```python
from build123d import *

# Parameters (mm, degrees)
F1_W     = 5.8
F1_H     = 2
F1_W_2   = 2
F2_DEPTH = 9
F3_DEPTH = 25
F4_R     = 1
F6_DEPTH = 7


with BuildPart() as f2:
    # F1 (on Top) → F2 (new body, symmetric)
    with BuildSketch(Plane.XY):
        with Locations((22.9, 1)):
            Rectangle(F1_W, F1_H)
        with Locations((26.8, 1)):
            Rectangle(F1_W_2, F1_H)
        Polygon((-29.8, 0), (-27.8, 0), (-27.8, 2), (-27.8, 27), (-27.8, 29), (-29.8, 29), align=None)
        Polygon((27.8, 29), (27.8, 27), (27.8, 2), (27.8, 0), (29.8, 0), (29.8, 29), align=None)
        Polygon((-27.8, 27), (-25.8, 27), (25.8, 27), (27.8, 27), (27.8, 29), (-27.8, 29), align=None)
        with Locations((-26.8, 1)):
            Rectangle(F1_W_2, F1_H)
        with Locations((-22.9, 1)):
            Rectangle(F1_W, F1_H)
    extrude(amount=F2_DEPTH, both=True)

    # F0 (on Front) → F3 (cut)
    with BuildSketch(Plane.XZ):
        with BuildLine():
            ThreePointArc((-24, 6.5), (-25.5, 5), (-24, 3.5))
            Line((-24, 3.5), (-24, 6.5))
        make_face()
        with BuildLine():
            Line((-24, 6.5), (-24, 3.5))
            ThreePointArc((-24, 3.5), (-22.9393398282, 3.9393398282), (-22.5, 5))
            ThreePointArc((-22.5, 5), (-22.9393398282, 6.0606601718), (-24, 6.5))
        make_face()
        with BuildLine():
            Line((-24, -6.5), (-24, -3.5))
            ThreePointArc((-24, -3.5), (-25.5, -5), (-24, -6.5))
        make_face()
        with BuildLine():
            ThreePointArc((-22.5, -5), (-22.9393398282, -3.9393398282), (-24, -3.5))
            Line((-24, -3.5), (-24, -6.5))
            ThreePointArc((-24, -6.5), (-22.9393398282, -6.0606601718), (-22.5, -5))
        make_face()
        with BuildLine():
            Line((24, 3), (24, 6))
            ThreePointArc((24, 6), (22.5, 4.5), (24, 3))
        make_face()
        with BuildLine():
            ThreePointArc((25.5, 4.5), (25.0606601718, 5.5606601718), (24, 6))
            Line((24, 6), (24, 3))
            ThreePointArc((24, 3), (25.0606601718, 3.4393398282), (25.5, 4.5))
        make_face()
        with BuildLine():
            Line((24, -3), (24, -6))
            ThreePointArc((24, -6), (25.0606601718, -5.5606601718), (25.5, -4.5))
            ThreePointArc((25.5, -4.5), (25.0606601718, -3.4393398282), (24, -3))
        make_face()
        with BuildLine():
            ThreePointArc((24, -3), (22.5, -4.5), (24, -6))
            Line((24, -6), (24, -3))
        make_face()
    extrude(amount=-F3_DEPTH, mode=Mode.SUBTRACT)

    # F4
    f4_edges = [f2.edges().sort_by_distance(p)[0] for p in [
        (-29.8, 0, 0),
        (29.8, 0, 0),
        (29.8, 29, 0),
        (-29.8, 29, 0),
    ]]
    fillet(f4_edges, radius=F4_R)

    # F5 (on face) → F6 (join)
    with BuildSketch(Plane.XZ.offset(-27)):
        with BuildLine():
            ThreePointArc((-6.4444444444, 0), (-9.4444444444, 3), (-12.4444444444, 0))
            Line((-12.4444444444, 0), (-6.4444444444, 0))
        make_face()
        with BuildLine():
            Line((-6.4444444444, 0), (-12.4444444444, 0))
            ThreePointArc((-12.4444444444, 0), (-9.4444444444, -3), (-6.4444444444, 0))
        make_face()
    extrude(amount=-F6_DEPTH)


solid = f2.part
```
Model file for the job. Use its own axes, mm. A direction names the side the tool comes from. Coordinates: 2 decimals unless noted, no trailing zeros. Loops run counter-clockwise (first coordinate to the right, second up) from the corner with the lowest first, then second, coordinate; pieces in that order, holes last. Notation, with made-up numbers: (18.5, 25) - (72.5, 25) arc R15 cw to (72.5, 32) - close; hole circle Ø10 at (55.25, -7.75). An arc over 180 degrees is marked (long way). Answer as a JSON object with one key per item and string values. Group by question number.
(1) Two-plate mould, pull along X, no slides. Class faces 1 (the face through (-6.447, 31.465, -0.132)), 2 (the face through (-9, 34, 0)), 3 (the face through (27.8, 15, 0)): released by +X, released by -X, zero draft, split by the parting line, or undercut.
(2) Flat gauge pins, fed straight in: pin 1 (1.5 mm diameter, centred on x = -7, z = 6, fed in from -Y); pin 2 (4 mm diameter, centred on x = 24, z = -1.5, fed in from +Y); pin 3 (5 mm diameter, centred on x = -1.5, y = 23.5, fed in from +Z). Where does each tip first touch, or does it go through?
(3) Cut at B-B (z = 0). Give the cut face in (x, y), then the cut area to 3 significant figures.
(4) Cut at A-A (y = 10). Give the cut face in (x, z), then the cut area to 3 significant figures.
(5) Cut at C-C (x = 4). Give the cut face in (y, z), then the cut area to 3 significant figures.
(6) Tool access for faces 4 (the face through (20, 1, 0)), 5 (the face through (-27.8, 14, 0)), 6 (the face through (-0.1, 27.5, -9)): list every direction of +Z, -Z, +X, -X, +Y, -Y with a clear straight run to the whole face (end or side of a thin tool).
(7) Cut at D-D (x = -7.5). Give the cut face in (y, z), then the cut area to 3 significant figures.
(8) Probe line 1 along X through (y, z) = (10, 2); line 2 along Y through (x, z) = (26, 6); line 3 along Y through (x, z) = (-14.5, 5.5). List the from-to ranges inside material, lowest first.
Geometry says:
{
 "1": {"face 1": "split by the parting line", "face 2": "zero draft", "face 3": "undercut"},
 "2": {"pin 1": "stops at y = 27", "pin 2": "stops at y = 29", "pin 3": "passes through"},
 "3": {"outline": "(-29.8, 1) arc R1 ccw to (-28.8, 0) - (-20, 0) - (-20, 2) - (-27.8, 2) - (-27.8, 27) - (27.8, 27) - (27.8, 2) - (20, 2) - (20, 0) - (28.8, 0) arc R1 ccw to (29.8, 1) - (29.8, 28) arc R1 ccw to (28.8, 29) - (-6.44, 29) - (-6.44, 34) - (-12.44, 34) - (-12.44, 29) - (-28.8, 29) arc R1 ccw to (-29.8, 28) - close", "area": "288 mm^2"},
 "4": {"outline": "(-29.8, -9) - (-27.8, -9) - (-27.8, 9) - (-29.8, 9) - close; (27.8, -9) - (29.8, -9) - (29.8, 9) - (27.8, 9) - close", "area": "72.0 mm^2"},
 "5": {"outline": "(27, -9) - (29, -9) - (29, 9) - (27, 9) - close", "area": "36.0 mm^2"},
 "6": {"face 4": "+Z, -Z, -Y", "face 5": "+Z, -Z", "face 6": "-Z, +X, -X, +Y, -Y"},
 "7": {"outline": "(27, -9) - (29, -9) - (29, -2.28) - (34, -2.28) - (34, 2.28) - (29, 2.28) - (29, 9) - (27, 9) - close", "area": "58.8 mm^2"},
 "8": {"line 1": "x = -29.8 to -27.8, 27.8 to 29.8", "line 2": "y = 0 to 2, 27 to 29", "line 3": "y = 27 to 29"}
}
